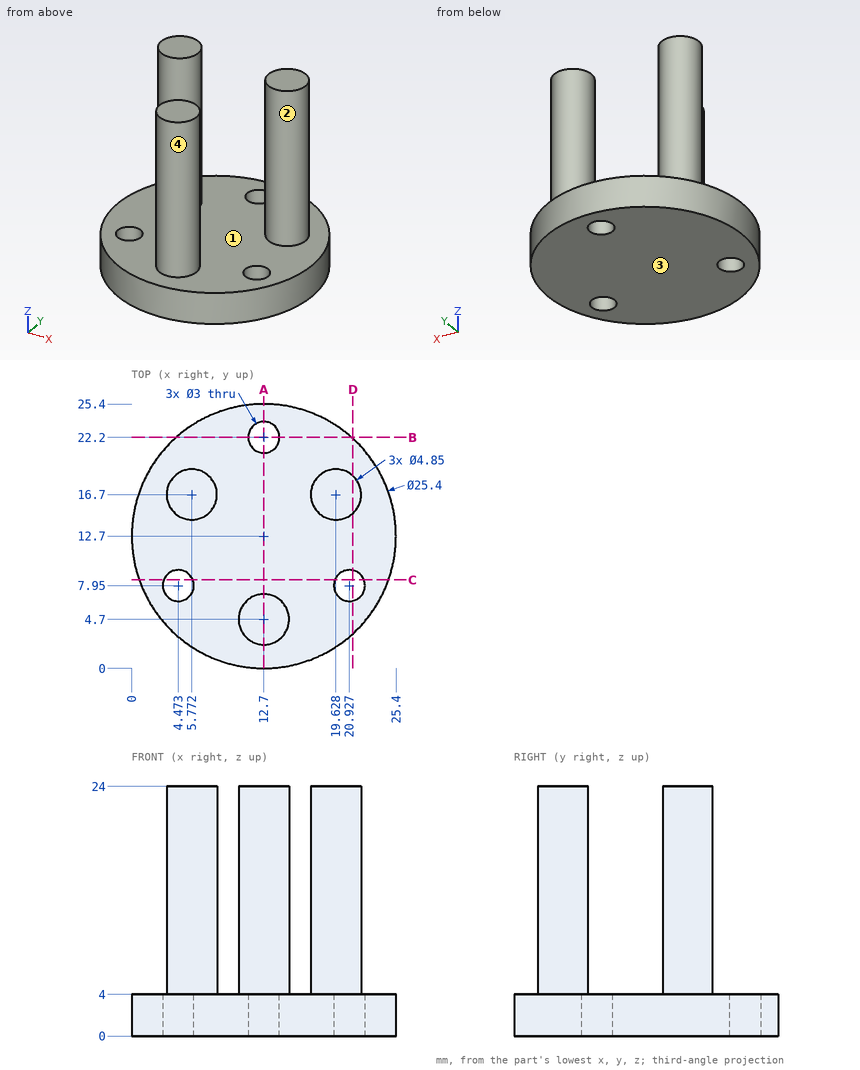
Geometry check sheet. Reference: drawing and pictorial views, mm from the part's lowest x, y, z. A direction names the side the tool comes from. Round coordinates to 2 decimals unless told otherwise and drop trailing zeros. Order: outer loops, then holes, each group sorted by start corner. A loop starts at its lowest first (then second) coordinate and runs counter-clockwise, first axis right, second up. Notation, with made-up numbers: (-21, -6.5) - (28, -6.5) arc R36 cw to (28, 29.5) - close; hole circle Ø4 at (18, 71). An arc over 180 degrees is marked (long way). Use a Markdown table: item, result. Add a question column.
1) Section check C-C (y = 8.5). Record the cut outline in (x, z) (1 decimal).
2) Thickness scan on line 1 along X through (y, z) = (7.5, 1.5); line 2 along Y through (x, z) = (12.7, 2.8); line 3 along Z through (x, y) = (5.25, 21). Record the ranges inside material, lowest first.
3) Set-up check for the marked faces 3 and 4: record each of +Z, -Z, +X, -X, +Y, -Y from which the full face is reachable in a straight line by a thin tool's end or side.
4) Mould release check, pull along Y, two halves, no side actions. Record for the marked faces 1 and 2: released by +Y, released by -Y, zero draft, split by the parting line, or undercut.
5) Section check D-D (x = 21.25). Record the cut outline in (y, z) (1 decimal).
6) Section check B-B (y = 22.2). Record the cut outline in (x, z).
7) Section check A-A (x = 12.7). Record the cut outline in (y, z) (3 decimals), then the cut area to 3 significant figures.
8) Gauge pin test, flat ends, axial feed: P1, Ø12, axis at x = 16, y = 19, coming from the +Z side; P2, Ø1, axis at x = 20, y = 13, coming from the +Z side; P3, Ø5, axis at x = 22.5, z = 9, coming from the -Y side; P4, Ø1, axis at y = 18.5, z = 11.5, coming from the +X side (1 decimal). Record the tip position at first contact, or that the pin passes through.
Established:
| question | item | result |
|---|---|---|
| 1 | outline | (0.7, 0) - (3.1, 0) - (3.1, 4) - (0.7, 4) - close; (5.9, 0) - (19.5, 0) - (19.5, 4) - (5.9, 4) - close; (22.3, 0) - (24.7, 0) - (24.7, 4) - (22.3, 4) - close |
| 2 | line 1 | 1.11 to 3.04, 5.9 to 19.5, 22.36 to 24.29 |
| 2 | line 2 | 0 to 20.7, 23.7 to 25.4 |
| 2 | line 3 | 0 to 4 |
| 3 | face 3 | -Z, +X, -X, +Y, -Y |
| 3 | face 4 | +Z |
| 4 | face 1 | zero draft |
| 4 | face 2 | split by the parting line |
| 5 | outline | (3.3, 0) - (6.5, 0) - (6.5, 4) - (3.3, 4) - close; (9.4, 0) - (22.1, 0) - (22.1, 4) - (18.5, 4) - (18.5, 24) - (14.9, 24) - (14.9, 4) - (9.4, 4) - close |
| 6 | outline | (4.27, 0) - (11.2, 0) - (11.2, 4) - (4.27, 4) - close; (14.2, 0) - (21.13, 0) - (21.13, 4) - (14.2, 4) - close |
| 7 | outline | (0, 0) - (20.7, 0) - (20.7, 4) - (7.125, 4) - (7.125, 24) - (2.275, 24) - (2.275, 4) - (0, 4) - close; (23.7, 0) - (25.4, 0) - (25.4, 4) - (23.7, 4) - close |
| 7 | area | 187 mm2 |
| 8 | P1 | z = 24 |
| 8 | P2 | z = 4 |
| 8 | P3 | y = 14.3 |
| 8 | P4 | x = 21.7 |
